```python
from build123d import *

# Parameters (mm, degrees)
SKETCH1_R           = 14.3
BOSS_EXTRUDE1_DEPTH = 5
SKETCH2_R           = 6.5
BOSS_EXTRUDE2_DEPTH = 20.5
SKETCH5_R           = 1.125
CUT_EXTRUDE1_DEPTH  = 15
SKETCH6_R           = 4.85
CUT_EXTRUDE2_DEPTH  = 25.5
SKETCH7_W           = 3.263473237
SKETCH7_H           = 32.347337023
SKETCH7_W_2         = 3.52826165
CUT_EXTRUDE5_DEPTH  = 10


with BuildPart() as part:
    # Sketch1 → Boss-Extrude1 (new body)
    with BuildSketch(Plane(origin=(0, 0, 0), x_dir=(1, 0, 0), z_dir=(0, 1, 0))):
        Circle(SKETCH1_R)
    extrude(amount=BOSS_EXTRUDE1_DEPTH)

    # Sketch2 → Boss-Extrude2 (add)
    with BuildSketch(Plane.XZ):
        Circle(SKETCH2_R)
    extrude(amount=BOSS_EXTRUDE2_DEPTH)

    # Sketch5 → Cut-Extrude1 (cut)
    with BuildSketch(Plane(origin=(0, 5, 0), x_dir=(1, 0, 0), z_dir=(0, 1, 0))):
        with Locations((0, -11.25)):
            Circle(SKETCH5_R)
        with Locations((0, 11.25)):
            Circle(SKETCH5_R)
    extrude(amount=-CUT_EXTRUDE1_DEPTH, mode=Mode.SUBTRACT)

    # Sketch6 → Cut-Extrude2 (cut)
    with BuildSketch(Plane.XZ.offset(20.5)):
        Circle(SKETCH6_R)
    extrude(amount=-CUT_EXTRUDE2_DEPTH, mode=Mode.SUBTRACT)

    # Sketch7 → Cut-Extrude5 (cut)
    with BuildSketch(Plane(origin=(0, 5, 0), x_dir=(1, 0, 0), z_dir=(0, 1, 0))):
        with Locations((13.631736618, 0.768402462)):
            Rectangle(SKETCH7_W, SKETCH7_H)
        with Locations((-13.764130825, 0.768402462)):
            Rectangle(SKETCH7_W_2, SKETCH7_H)
    extrude(amount=-CUT_EXTRUDE5_DEPTH, mode=Mode.SUBTRACT)


solid = part.part
```
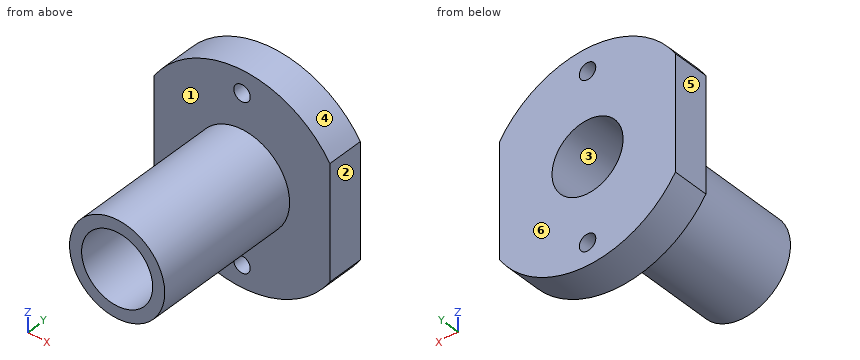
Input: part model. Units: mm. Frame: model coordinates. Face numbers are marked on the shaded views. A direction names the side the tool comes from. Coordinates: 2 decimals unless noted, no trailing zeros. Write each loop counter-clockwise with the first axis right and the second up, starting at its lowest first coordinate (ties: lowest second). Pieces come first, ordered by that corner, then holes. Notation, with made-up numbers: (8.25, 1.5) - (17.25, 1.5) arc R18 ccw to (17.25, 22.5) - close; hole circle Ø9 at (42, -30). An arc over 180 degrees is marked (long way). Put each result on its own line as item: value. Start each with the question number.
1) Contact query for flat-ended pins moving along their axis: pin 1 (4 mm diameter, centred on x = 0.5, z = 1.5, fed in from -Y) (3 decimals); pin 2 (8 mm diameter, centred on x = 6.5, y = -10, fed in from -Z). Output: stop coordinate, or through.
2) Cut plane B-B (z = 0). Return the cut outline in (x, y), plus the area to 3 significant figures.
3) Cut plane A-A (x = 0). Return the cut outline in (y, z) (3 decimals), plus the area to 3 significant figures.
4) Ray query, L1, parallel to Z at x = 0, y = 3.3 (3 decimals); L2, parallel to Z at x = -1, y = 3.25 (3 decimals); L3, parallel to Z at x = 0, y = -8.75. Return the intervals inside material, ascending.
5) Mould query, pull axis X, two halves, no side actions, for the marked faces 3, 4, 5 and 6. Classes: pulls with the +X half, pulls with the -X half, needs draft (parallel to the pull), parting line crosses it, or undercut.
6) Reachability of the marked faces 1 and 2 from +Z, -Z, +X, -X, +Y, -Y: full face, straight path, thin tool, end or side. Return the list, or none.
7) Cut plane D-D (z = -11.75). Return the cut outline in (x, y), plus the area to 3 significant figures.
8) Cut plane C-C (y = -1.5). Return the cut outline in (x, z).
Resolved:
1. pin 1: passes through
1. pin 2: stops at z = -6
2. outline: (-12, 0) - (-6.5, 0) - (-6.5, -20.5) - (-4.85, -20.5) - (-4.85, 5) - (-12, 5) - close; (4.85, -20.5) - (6.5, -20.5) - (6.5, 0) - (12, 0) - (12, 5) - (4.85, 5) - close
2. area: 139 mm2
3. outline: (-20.5, -6.5) - (0, -6.5) - (0, -10.125) - (5, -10.125) - (5, -4.85) - (-20.5, -4.85) - close; (-20.5, 4.85) - (5, 4.85) - (5, 10.125) - (0, 10.125) - (0, 6.5) - (-20.5, 6.5) - close; (0, -14.3) - (5, -14.3) - (5, -12.375) - (0, -12.375) - close; (0, 12.375) - (5, 12.375) - (5, 14.3) - (0, 14.3) - close
3. area: 140 mm2
4. L1: z = -14.3 to -12.375, -10.125 to -4.85, 4.85 to 10.125, 12.375 to 14.3
4. L2: z = -14.265 to -11.765, -10.735 to -4.746, 4.746 to 10.735, 11.765 to 14.265
4. L3: z = -6.5 to -4.85, 4.85 to 6.5
5. face 3: undercut
5. face 4: parting line crosses it
5. face 5: pulls with the -X half
5. face 6: needs draft
6. face 1: -Y
6. face 2: +Z, -Z, +X, +Y, -Y
7. outline: (-8.15, 0) - (-1.01, 0) - (-1.01, 5) - (-8.15, 5) - close; (1.01, 0) - (8.15, 0) - (8.15, 5) - (1.01, 5) - close
7. area: 71.4 mm2
8. outline: circle Ø13 at (0, 0); hole circle Ø9.7 at (0, 0)
